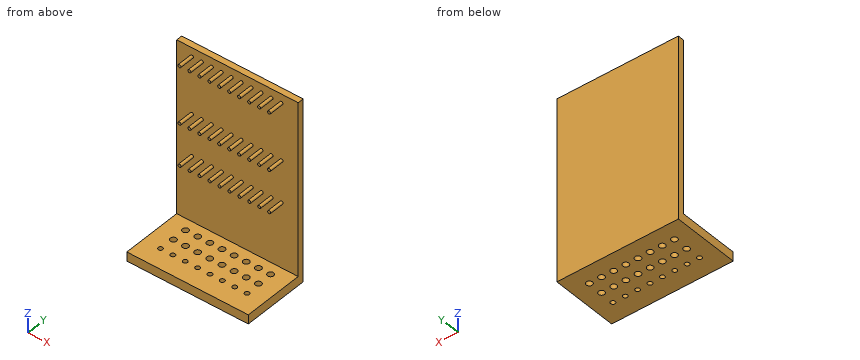
```python
from build123d import *

# Parameters (mm, degrees)
F0_W      = 101.6
F0_H      = 152.4
F1_DEPTH  = 5.08
F2_W      = 101.6
F2_H      = 7.62
F3_DEPTH  = 50.8
F4_R      = 2.54
F5_DEPTH  = 25.4
F6_R      = 2.54
F7_DEPTH  = 25.4
F8_R      = 1.905
F9_DEPTH  = 25.4
F10_R     = 1.27
F11_DEPTH = 12.7
F12_R     = 1.27
F13_DEPTH = 12.7
F14_R     = 1.27
F15_DEPTH = 12.7


with BuildPart() as f1:
    # F0 (on Front) → F1 (new body)
    with BuildSketch(Plane.XZ):
        with Locations((-9.830583, 25.110631)):
            Rectangle(F0_W, F0_H)
    extrude(amount=F1_DEPTH)

    # F2 (on face) → F3 (join)
    with BuildSketch(Plane.XZ.offset(5.08)):
        with Locations((-9.830583, -47.279369)):
            Rectangle(F2_W, F2_H)
    extrude(amount=F3_DEPTH)

    # F4 (on face) → F5 (cut)
    with BuildSketch(Plane.XY.offset(-43.469369)):
        with Locations((-45.390583, -14.613039)):
            Circle(F4_R)
        with Locations((-35.230583, -14.613039)):
            Circle(F4_R)
        with Locations((-25.070583, -14.613039)):
            Circle(F4_R)
        with Locations((-14.910583, -14.613039)):
            Circle(F4_R)
        with Locations((-4.750583, -14.613039)):
            Circle(F4_R)
        with Locations((5.409417, -14.613039)):
            Circle(F4_R)
        with Locations((15.569417, -14.613039)):
            Circle(F4_R)
        with Locations((25.729417, -14.613039)):
            Circle(F4_R)
    extrude(amount=-F5_DEPTH, mode=Mode.SUBTRACT)

    # F6 (on face) → F7 (cut)
    with BuildSketch(Plane.XY.offset(-43.469369)):
        with Locations((-45.390583, -27.030999)):
            Circle(F6_R)
        with Locations((-35.230583, -27.030999)):
            Circle(F6_R)
        with Locations((-25.070583, -27.030999)):
            Circle(F6_R)
        with Locations((-14.910583, -27.030999)):
            Circle(F6_R)
        with Locations((-4.750583, -27.030999)):
            Circle(F6_R)
        with Locations((5.409417, -27.030999)):
            Circle(F6_R)
        with Locations((15.569417, -27.030999)):
            Circle(F6_R)
        with Locations((25.729417, -27.030999)):
            Circle(F6_R)
    extrude(amount=-F7_DEPTH, mode=Mode.SUBTRACT)

    # F8 (on face) → F9 (cut)
    with BuildSketch(Plane.XY.offset(-43.469369)):
        with Locations((26.364417, -39.353926)):
            Circle(F8_R)
        with Locations((16.022989, -39.353926)):
            Circle(F8_R)
        with Locations((5.68156, -39.353926)):
            Circle(F8_R)
        with Locations((-4.659868, -39.353926)):
            Circle(F8_R)
        with Locations((-15.001297, -39.353926)):
            Circle(F8_R)
        with Locations((-25.342725, -39.353926)):
            Circle(F8_R)
        with Locations((-35.684154, -39.353926)):
            Circle(F8_R)
        with Locations((-46.025583, -39.353926)):
            Circle(F8_R)
    extrude(amount=-F9_DEPTH, mode=Mode.SUBTRACT)

    # F10 (on face) → F11 (join)
    with BuildSketch(Plane.XZ.offset(5.08)):
        with Locations((-47.930583, 93.943223)):
            Circle(F10_R)
        with Locations((-39.605027, 93.943223)):
            Circle(F10_R)
        with Locations((-31.279471, 93.943223)):
            Circle(F10_R)
        with Locations((-22.953916, 93.943223)):
            Circle(F10_R)
        with Locations((-14.62836, 93.943223)):
            Circle(F10_R)
        with Locations((-6.302805, 93.943223)):
            Circle(F10_R)
        with Locations((2.022751, 93.943223)):
            Circle(F10_R)
        with Locations((10.348306, 93.943223)):
            Circle(F10_R)
        with Locations((18.673862, 93.943223)):
            Circle(F10_R)
        with Locations((26.999417, 93.943223)):
            Circle(F10_R)
    extrude(amount=F11_DEPTH)

    # F12 (on face) → F13 (join)
    with BuildSketch(Plane.XZ.offset(5.08)):
        with Locations((-47.930583, 46.068911)):
            Circle(F12_R)
        with Locations((-39.605027, 46.068911)):
            Circle(F12_R)
        with Locations((-31.279471, 46.068911)):
            Circle(F12_R)
        with Locations((-22.953916, 46.068911)):
            Circle(F12_R)
        with Locations((-14.62836, 46.068911)):
            Circle(F12_R)
        with Locations((-6.302805, 46.068911)):
            Circle(F12_R)
        with Locations((2.022751, 46.068911)):
            Circle(F12_R)
        with Locations((10.348306, 46.068911)):
            Circle(F12_R)
        with Locations((18.673862, 46.068911)):
            Circle(F12_R)
        with Locations((26.999417, 46.068911)):
            Circle(F12_R)
    extrude(amount=F13_DEPTH)

    # F14 (on face) → F15 (join)
    with BuildSketch(Plane.XZ.offset(5.08)):
        with Locations((-47.791654, 11.04094)):
            Circle(F14_R)
        with Locations((-39.466098, 11.04094)):
            Circle(F14_R)
        with Locations((-31.140543, 11.04094)):
            Circle(F14_R)
        with Locations((-22.814987, 11.04094)):
            Circle(F14_R)
        with Locations((-14.489432, 11.04094)):
            Circle(F14_R)
        with Locations((-6.163876, 11.04094)):
            Circle(F14_R)
        with Locations((2.161679, 11.04094)):
            Circle(F14_R)
        with Locations((10.487235, 11.04094)):
            Circle(F14_R)
        with Locations((18.812791, 11.04094)):
            Circle(F14_R)
        with Locations((27.138346, 11.04094)):
            Circle(F14_R)
    extrude(amount=F15_DEPTH)


solid = f1.part
```
Design review of the part built by this model. Coordinates are the model's own, in mm. Give positions to 0.01 mm unless a question says otherwise; leave off trailing zeros. Write each loop counter-clockwise with the first axis right and the second up, starting at its lowest first coordinate (ties: lowest second). Pieces come first, ordered by that corner, then holes.
(1) Add section B-B (z = 29.5). Give the boundary of the cut face in (x, y), and give its area (3 significant figures).
Checked values:
outline: (-60.63, -5.08) - (40.97, -5.08) - (40.97, 0) - (-60.63, 0) - close
area: 516 mm2
(2) Add section A-A (y = -9). Give the number of separate pieces and of enclosed holes in the cut face, and give its area (3 significant figures).
Checked values:
separate pieces: 31
enclosed holes: 0
area: 926 mm2
(3) Clearance check with flat-ended pins moving along their axes: pin 1 Ø3 at (x, y) = (-4.75, -27.03) entering from +Z; pin 2 Ø3 at (x, z) = (-31, 45.5) entering from -Y; pin 3 Ø12 at (x, z) = (-49, 27.5) entering from -Y; pin 4 Ø6 at (x, y) = (25.73, -27.03) entering from +Z. State where each tip first meets the part, or that it passes through.
Checked values:
pin 1: passes through
pin 2: stops at y = -17.78
pin 3: stops at y = -5.08
pin 4: stops at z = -43.47
(4) Add section C-C (y = -21). Give the boundary of the cut face in (x, z), and give its area (3 significant figures).
Checked values:
outline: (-60.63, -51.09) - (40.97, -51.09) - (40.97, -43.47) - (-60.63, -43.47) - close
area: 774 mm2
(5) Wall thickness on line 1 along Y through (x, z) = (-55.5, -35); line 2 along Z through (x, y) = (-5.5, -19): over which ranges is each line inside the solid? List them lowest first.
Checked values:
line 1: y = -5.08 to 0
line 2: z = -51.09 to -43.47
